Can you work these out from the model? Positions are in its coordinate system, mm. A direction names the side the tool comes from. Coordinates: 2 decimals unless noted, no trailing zeros. Loops run counter-clockwise (first coordinate to the right, second up) from the corner with the lowest first, then second, coordinate; pieces in that order, holes last.
```python
from build123d import *

# Parameters (mm, degrees)
F0_W     = 371.475
F0_H     = 44.45
F1_DEPTH = 19.05
F2_W     = 6.35
F2_H     = 11.1125
F3_DEPTH = 371.476
F4_SIZE2 = 3.175
F4_SIZE  = 1.5875
F6_DEPTH = 19.051


with BuildPart() as f1:
    # F0 (on Front) → F1 (new body)
    with BuildSketch(Plane.XZ):
        Rectangle(F0_W, F0_H)
    extrude(amount=F1_DEPTH)

    # F2 (on face) → F3 (cut, through all)
    with BuildSketch(Plane(origin=(-185.7375, 0, 0), x_dir=(0, -1, 0), z_dir=(-1, 0, 0))):
        with Locations((9.525, 16.66875)):
            Rectangle(F2_W, F2_H)
    extrude(amount=-F3_DEPTH, mode=Mode.SUBTRACT)

    # F4
    f4_edges = [f1.edges().sort_by_distance(p)[0] for p in [
        (0, -19.05, 22.225),
    ]]
    chamfer(f4_edges, length=F4_SIZE, length2=F4_SIZE2)

    # F5 (on face) → F6 (cut, through all)
    with BuildSketch(Plane(origin=(0, 0, 0), x_dir=(-1, 0, 0), z_dir=(0, 1, 0))):
        Polygon((-185.7375, 22.225), (-185.7375, -22.225), (-141.2875, 22.225), align=None)
        Polygon((141.2875, 22.225), (185.7375, -22.225), (185.7375, 22.225), align=None)
    extrude(amount=-F6_DEPTH, mode=Mode.SUBTRACT)


solid = f1.part
```
(1) I'm going to push flat-ended pins straight in: pin 1 (1.9 mm diameter, centred on x = -18.5, y = -10.5, fed in from +Z); pin 2 (10 mm diameter, centred on y = -5, z = -16, fed in from -X); pin 3 (10 mm diameter, centred on y = -6.5, z = -13, fed in from +X). Where does each tip first touch, or does it pass through?
Check values:
pin 1: stops at z = 11.11
pin 2: stops at x = -184.51
pin 3: stops at x = 181.51
(2) I want a section at C-C on z = -8.5. Write out the boundary of the cut face in (x, y), then the cut area to 3 significant figures.
Check values:
outline: (-172.01, -19.05) - (172.01, -19.05) - (172.01, 0) - (-172.01, 0) - close
area: 6,550 mm2
(3) If I drill on probe 1 along Y at (x, z) = (-125, 16.5); probe 2 along Z at (x, y) = (-58.5, -9) (1 decimal); probe 3 along Z at (x, y) = (153, -3) (1 decimal), over which ranges is the centre line in solid material (lowest first)?
Check values:
probe 1: y = -19.05 to -12.7, -6.35 to 0
probe 2: z = -22.2 to 11.1
probe 3: z = -22.2 to 10.5
(4) I want a section at B-B on y = -3. Write out the boundary of the cut face in (x, z) (1 decimal), then the cut area to 3 significant figures.
Check values:
outline: (-185.7, -22.2) - (185.7, -22.2) - (141.3, 22.2) - (-141.3, 22.2) - close
area: 14,500 mm2
(5) If we mould it in two halves opening along Y, with no side actions, what happens to faces 3 (the flat face through (-2, -6.35, 17)), 4 (the flat face through (-3, -9, -22.225)), 5 (the flat face through (-3, -19.05, -1))? For each: released by +Y, released by -Y, zero draft, split by the parting line, or undercut.
Check values:
face 3: undercut
face 4: zero draft
face 5: released by -Y
(6) Which directions (+Z, -Z, +X, -X, +Y, -Y) give clear straight access to the entire face, cutting with the end or side of a thin tool? Please do faces 1 (the flat face through (-2, -12.7, 17)), 2 (the flat face through (-3, 0, 0)).
Check values:
face 1: +Z, +X, -X
face 2: +Z, -Z, +X, -X, +Y
